Design review of the part built by this model. Coordinates are the model's own, in mm. A direction names the side the tool comes from. Round coordinates to 2 decimals unless told otherwise and drop trailing zeros. Loops run counter-clockwise (first coordinate to the right, second up) from the corner with the lowest first, then second, coordinate; pieces in that order, holes last. Notation, with made-up numbers: (-3, 71) - (45, 71) arc R21 cw to (45, 109) - close; hole circle Ø8 at (-30, 1). An arc over 180 degrees is marked (long way). Return JSON: item names as keys, results as strings. Group by question number.
(1) We need section A-A, the plane y = -29. Write out the cut boundary in (x, z).
(2) Wall thickness on L1, parallel to X at y = -85, z = -2.75; L2, parallel to Y at x = 2, z = 11.25; L3, parallel to X at y = -37, z = 3.25: over which ranges is each line inside the solid? List them lowest first. Write a range as [from, to].
(3) Clearance check with flat-ended pins moving along their axes: pin 1 (10 mm diameter, centred on x = 3, y = -49.5, fed in from +Z); pin 2 (6.5 mm diameter, centred on y = -135.5, z = 0.5, fed in from -X); pin 3 (10 mm diameter, centred on y = -132, z = -5.5, fed in from +X); pin 4 (8 mm diameter, centred on x = 7.5, z = -4.5, fed in from -Y). State where each tip first meets the part, or that it passes through.
(4) For faces 1 (the flat face through (5.3, -200, 0.2)), 2 (the cylindrical face through (5.19, -223.71, -9.98)), 3 (the flat face through (-5, -104, 0)), 4 (the flat face through (5, -104, 0)), list the 3-axis set-ups (+Z, -Z, +X, -X, +Y, -Y) from which the entire face can be reached by the end or side of a thin tool; tool diameter is ignored.
from build123d import *

# Parameters (mm, degrees)
F1_DEPTH    = 200
F2_R        = 11.25
F3_DEPTH    = 50
F4_R        = 12.5
F5_DEPTH    = 3
F6_R        = 1
F7_R        = 5
F8_T1_DEPTH = 57.7361444178
F8_T3_DEPTH = 57.7361444178
F8_T5_DEPTH = 57.7361444178
F8_T7_DEPTH = 57.7361444178
F8_T9_DEPTH = 57.7361444178
F9_T1_DEPTH = 11.6621406423
F9_T3_DEPTH = 11.6621406423
F9_T5_DEPTH = 11.6621406423
F9_T7_DEPTH = 11.6621406423


# Not quite as in the source:
# - a fillet or chamfer that OpenCascade refuses, or shapes differently, is made with other operations: its cross-section is extruded or revolved along the edge and cut away or added


with BuildPart() as f1:
    # F0 (on Front) → F1 (new body)
    with BuildSketch(Plane.XZ):
        with BuildLine():
            ThreePointArc((2.5000000636, -4.3301269822), (4.3301270373, -2.4999999682), (5, 0))
            ThreePointArc((5, 0), (4.3301270373, 2.4999999682), (2.5000000636, 4.3301269822))
            ThreePointArc((2.5000000636, 4.3301269822), (1.215e-07, 5), (-2.4999998532, 4.3301271037))
            ThreePointArc((-2.4999998532, 4.3301271037), (-4.3301269765, 2.5000000734), (-5, 0))
            ThreePointArc((-5, 0), (-4.3301270351, -2.4999999721), (-2.5000000559, -4.3301269867))
            ThreePointArc((-2.5000000559, -4.3301269867), (4.5e-09, -5), (2.5000000636, -4.3301269822))
        make_face()
        with BuildLine():
            Line((5, -2.8867513459), (5, 0))
            ThreePointArc((5, 0), (4.3301270373, -2.4999999682), (2.5000000636, -4.3301269822))
            Line((2.5000000636, -4.3301269822), (5, -2.8867513459))
        make_face()
        with BuildLine():
            ThreePointArc((2.5000000636, 4.3301269822), (4.3301270373, 2.4999999682), (5, 0))
            Line((5, 0), (5, 2.8867513459))
            Line((5, 2.8867513459), (2.5000000636, 4.3301269822))
        make_face()
        with BuildLine():
            ThreePointArc((-2.4999998532, 4.3301271037), (1.215e-07, 5), (2.5000000636, 4.3301269822))
            Line((2.5000000636, 4.3301269822), (0, 5.7735026919))
            Line((0, 5.7735026919), (-2.4999998532, 4.3301271037))
        make_face()
        with BuildLine():
            Line((0, -5.7735026919), (2.5000000636, -4.3301269822))
            ThreePointArc((2.5000000636, -4.3301269822), (4.5e-09, -5), (-2.5000000559, -4.3301269867))
            Line((-2.5000000559, -4.3301269867), (0, -5.7735026919))
        make_face()
        with BuildLine():
            ThreePointArc((-5, 0), (-4.3301269765, 2.5000000734), (-2.4999998532, 4.3301271037))
            Line((-2.4999998532, 4.3301271037), (-5, 2.8867513459))
            Line((-5, 2.8867513459), (-5, 0))
        make_face()
        with BuildLine():
            Line((-5, -2.8867513459), (-2.5000000559, -4.3301269867))
            ThreePointArc((-2.5000000559, -4.3301269867), (-4.3301270351, -2.4999999721), (-5, 0))
            Line((-5, 0), (-5, -2.8867513459))
        make_face()
    extrude(amount=F1_DEPTH)

    # F2 (on face) → F3 (join)
    with BuildSketch(Plane.XZ.offset(200)):
        Circle(F2_R)
    extrude(amount=F3_DEPTH)

    # F4 (on face) → F5 (join)
    with BuildSketch(Plane(origin=(0, -200, 0), x_dir=(-1, 0, 0), z_dir=(0, 1, 0))):
        Circle(F4_R)
    extrude(amount=-F5_DEPTH)

    # F6
    f6_edges = [f1.edges().sort_by_distance(p)[0] for p in [
        (12.5, -203, 0),
        (12.5, -200, 0),
    ]]
    fillet(f6_edges, radius=F6_R)

    # F7
    f7_edges = [f1.edges().sort_by_distance(p)[0] for p in [
        (-11.25, -250, 0),
    ]]
    fillet(f7_edges, radius=F7_R)

    # F8: chamfer of 2 x 10 on 6 edges, made by hand

    # F8_s2 → F8_t1 (cut)
    with BuildSketch(Plane.XY.offset(-28.8680722089)):
        Polygon((5, -10), (3, 0), (5, 0), align=None)
        Polygon((-5, -10), (-3, 0), (-5, 0), align=None)
    extrude(amount=F8_T1_DEPTH, mode=Mode.SUBTRACT)

    # F8_s4 → F8_t3 (cut)
    with BuildSketch(Plane(origin=(25.0004838912, 0, -14.4340361045), x_dir=(0, 1, 0), z_dir=(-0.8660254038, 0, 0.5))):
        Polygon((-10, -5), (0, -3), (0, -5), align=None)
    extrude(amount=F8_T3_DEPTH, mode=Mode.SUBTRACT)

    # F8_s6 → F8_t5 (cut)
    with BuildSketch(Plane(origin=(25.0004838912, 0, 14.4340361045), x_dir=(0, 1, 0), z_dir=(-0.8660254038, 0, -0.5))):
        Polygon((-10, -5), (0, -3), (0, -5), align=None)
    extrude(amount=F8_T5_DEPTH, mode=Mode.SUBTRACT)

    # F8_s8 → F8_t7 (cut)
    with BuildSketch(Plane(origin=(-25.0004838912, 0, 14.4340361045), x_dir=(0, 1, 0), z_dir=(0.8660254038, 0, -0.5))):
        Polygon((-10, -5), (0, -3), (0, -5), align=None)
    extrude(amount=F8_T7_DEPTH, mode=Mode.SUBTRACT)

    # F8_s10 → F8_t9 (cut)
    with BuildSketch(Plane(origin=(-25.0004838912, 0, -14.4340361045), x_dir=(0, 1, 0), z_dir=(0.8660254038, 0, 0.5))):
        Polygon((-10, -5), (0, -3), (0, -5), align=None)
    extrude(amount=F8_T9_DEPTH, mode=Mode.SUBTRACT)

    # F9: fillet of radius 2 on 5 edges, made by hand

    # F9_s2 → F9_t1 (cut)
    with BuildSketch(Plane.XY.offset(-5.8310703212)):
        with BuildLine():
            ThreePointArc((3.3215535459, -1.6077677297), (2.6283700058, -0.4533157173), (1.3603921946, 0))
            Line((1.3603921946, 0), (3, 0))
            Line((3, 0), (3.3215535459, -1.6077677297))
        make_face()
        with BuildLine():
            ThreePointArc((-3.3215535459, -1.6077677297), (-2.6283700058, -0.4533157173), (-1.3603921946, 0))
            Line((-1.3603921946, 0), (-3, 0))
            Line((-3, 0), (-3.3215535459, -1.6077677297))
        make_face()
    extrude(amount=F9_T1_DEPTH, mode=Mode.SUBTRACT)

    # F9_s4 → F9_t3 (cut)
    with BuildSketch(Plane(origin=(5.0498550294, 0, 2.9155351606), x_dir=(0, 1, 0), z_dir=(-0.8660254038, 0, -0.5))):
        with BuildLine():
            ThreePointArc((-1.6077677297, -3.3215535459), (-0.4533157173, -2.6283700058), (0, -1.3603921946))
            Line((0, -1.3603921946), (0, -3))
            Line((0, -3), (-1.6077677297, -3.3215535459))
        make_face()
    extrude(amount=F9_T3_DEPTH, mode=Mode.SUBTRACT)

    # F9_s6 → F9_t5 (cut)
    with BuildSketch(Plane(origin=(-5.0498550294, 0, 2.9155351606), x_dir=(0, 1, 0), z_dir=(0.8660254038, 0, -0.5))):
        with BuildLine():
            ThreePointArc((-1.6077677297, -3.3215535459), (-0.4533157173, -2.6283700058), (0, -1.3603921946))
            Line((0, -1.3603921946), (0, -3))
            Line((0, -3), (-1.6077677297, -3.3215535459))
        make_face()
    extrude(amount=F9_T5_DEPTH, mode=Mode.SUBTRACT)

    # F9_s8 → F9_t7 (cut)
    with BuildSketch(Plane(origin=(5.0498550294, 0, -2.9155351606), x_dir=(0, 1, 0), z_dir=(-0.8660254038, 0, 0.5))):
        with BuildLine():
            ThreePointArc((-1.6077677297, -3.3215535459), (-0.4533157173, -2.6283700058), (0, -1.3603921946))
            Line((0, -1.3603921946), (0, -3))
            Line((0, -3), (-1.6077677297, -3.3215535459))
        make_face()
    extrude(amount=F9_T7_DEPTH, mode=Mode.SUBTRACT)


solid = f1.part
Solutions:
{
 "1": {"outline": "(-5, -2.89) - (0, -5.77) - (5, -2.89) - (5, 2.89) - (0, 5.77) - (-5, 2.89) - close"},
 "2": {"L1": "[-5, 5]", "L2": "[-203, -200]", "L3": "[-4.37, 4.37]"},
 "3": {"pin 1": "z = 5.77", "pin 2": "x = -5", "pin 3": "x = 5", "pin 4": "y = -250"},
 "4": {"face 1": "+Y", "face 2": "-Y", "face 3": "+Z, -Z, -X, +Y", "face 4": "+Z, -Z, +X, +Y"}
}
